```python
from build123d import *

# Parameters (mm, degrees)
F1_DEPTH  = 25.4
F4_SIZE   = 2.286
F5_SIZE   = 3.048
F3_W      = 3.048
F3_H      = 2.286
F6_DEPTH  = 20.066
F7_R      = 8.255
F9_DEPTH  = 25.4
F8_R      = 2.413
F10_DEPTH = 25.4
F11_SIZE  = 1.27
F13_R     = 12.065
F14_DEPTH = 6.35


with BuildPart() as f1:
    # F0 (on Front) → F1 (new body)
    with BuildSketch(Plane.XZ):
        Polygon((18.037553, -0.029708), (9.044504, 15.606125), (-8.993048, 15.635833), (-18.037553, 0.029708), (-9.044504, -15.606125), (8.993048, -15.635833), align=None)
    extrude(amount=F1_DEPTH)

    # F4
    f4_edges = [f1.edges().sort_by_distance(p)[0] for p in [
        (13.541028, 0, 7.788208),
        (0.025728, 0, 15.620979),
        (-13.515301, 0, 7.83277),
        (-13.541028, 0, -7.788208),
        (-0.025728, 0, -15.620979),
        (13.515301, 0, -7.83277),
    ]]
    chamfer(f4_edges, length=F4_SIZE)

    # F5
    f5_edges = [f1.edges().sort_by_distance(p)[0] for p in [
        (13.541028, -25.4, 7.788208),
        (0.025728, -25.4, 15.620979),
        (-13.515301, -25.4, 7.83277),
        (-13.541028, -25.4, -7.788208),
        (-0.025728, -25.4, -15.620979),
        (13.515301, -25.4, -7.83277),
    ]]
    chamfer(f5_edges, length=F5_SIZE)

    # F3 (on offset) → F6 (join)
    with BuildSketch(Plane.XZ.offset(2.286)):
        with Locations((18.87098, 0)):
            Rectangle(F3_W, F3_H)
        Polygon((9.207623, 18.234071), (7.683623, 15.594425), (9.663357, 14.451425), (11.187357, 17.091071), align=None)
        Polygon((-11.187357, 17.091071), (-9.663357, 14.451425), (-7.683623, 15.594425), (-9.207623, 18.234071), align=None)
        with Locations((-18.87098, 0)):
            Rectangle(F3_W, F3_H)
        Polygon((-9.207623, -18.234071), (-7.683623, -15.594425), (-9.663357, -14.451425), (-11.187357, -17.091071), align=None)
        Polygon((11.187357, -17.091071), (9.663357, -14.451425), (7.683623, -15.594425), (9.207623, -18.234071), align=None)
    extrude(amount=F6_DEPTH)

    # F7 (on Front) → F9 (join)
    with BuildSketch(Plane.XZ):
        Circle(F7_R)
    extrude(amount=-F9_DEPTH)

    # F8 (on Front) → F10 (cut)
    with BuildSketch(Plane.XZ):
        Circle(F8_R)
    extrude(amount=-F10_DEPTH, mode=Mode.SUBTRACT)

    # F11
    f11_edges = [f1.edges().sort_by_distance(p)[0] for p in [
        (8.255, 12.7, 0),
        (-8.255, 0, 0),
        (-8.255, 25.4, 0),
    ]]
    chamfer(f11_edges, length=F11_SIZE)

    # F13 (on offset) → F14 (cut)
    with BuildSketch(Plane.XZ.offset(25.4)):
        Circle(F13_R)
    extrude(amount=-F14_DEPTH, mode=Mode.SUBTRACT)


solid = f1.part
```
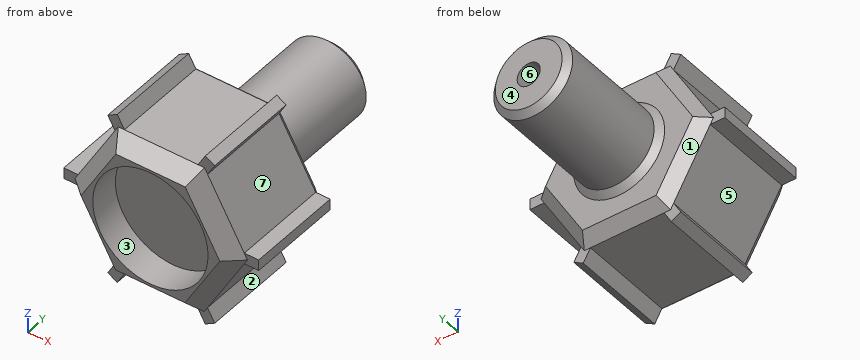
Part model, mm, in its own coordinate system. Face numbers are marked on the shaded views. A direction names the side the tool comes from. Round coordinates to 2 decimals unless told otherwise and drop trailing zeros. Loops run counter-clockwise (first coordinate to the right, second up) from the corner with the lowest first, then second, coordinate; pieces in that order, holes last.
1. Slice it at B-B (x = 0). Give the cut face in (y, z) (3 decimals).
Solutions:
outline: (-25.4, -12.573) - (-22.352, -15.621) - (-2.286, -15.621) - (0, -13.335) - (0, -9.525) - (1.27, -8.255) - (24.13, -8.255) - (25.4, -6.985) - (25.4, -2.413) - (0, -2.413) - (0, 2.413) - (25.4, 2.413) - (25.4, 6.985) - (24.13, 8.255) - (1.27, 8.255) - (0, 9.525) - (0, 13.335) - (-2.286, 15.621) - (-22.352, 15.621) - (-25.4, 12.573) - (-25.4, 12.065) - (-19.05, 12.065) - (-19.05, -12.065) - (-25.4, -12.065) - close
2. Drill centre lines: line 1 along Y through (x, z) = (4, 12); line 2 along Z through (x, y) = (0, 6.5) (3 decimals); line 3 along Y through (x, z) = (1, -3). Where is each one in solid material? Low to high.
Solutions:
line 1: y = -25.4 to 0
line 2: z = -8.255 to -2.413, 2.413 to 8.255
line 3: y = -19.05 to 25.4
3. Two-plate mould, pull along X, no slides. Class the marked faces 1, 2, 3 and 4: pulls with the +X half, pulls with the -X half, needs draft (parallel to the pull), parting line crosses it, or undercut.
Solutions:
face 1: pulls with the -X half
face 2: pulls with the +X half
face 3: undercut
face 4: needs draft
4. Slice it at A-A (y = -20). Give the cut face in (x, z) (3 decimals), and give its area (3 significant figures).
Solutions:
outline: (-20.395, -1.143) - (-17.363, -1.143) - (-9.686, -14.491) - (-11.187, -17.091) - (-9.208, -18.234) - (-7.692, -15.608) - (7.706, -15.634) - (9.208, -18.234) - (11.187, -17.091) - (9.671, -14.465) - (17.392, -1.143) - (20.395, -1.143) - (20.395, 1.143) - (17.363, 1.143) - (9.686, 14.491) - (11.187, 17.091) - (9.208, 18.234) - (7.692, 15.608) - (-7.706, 15.634) - (-9.208, 18.234) - (-11.187, 17.091) - (-9.671, 14.465) - (-17.392, 1.143) - (-20.395, 1.143) - close; hole circle Ø24.13 at (0, 0)
area: 425 mm2
5. Slice it at C-C (y = 11.5). Give the cut face in (x, z) (3 decimals), and give its area (3 significant figures).
Solutions:
outline: circle Ø16.51 at (0, 0); hole circle Ø4.826 at (0, 0)
area: 196 mm2
6. 3-axis set-ups, long thin cutter, end or side, ignore diameter. For the marked faces 5, 6 and 7: which of +Z, -Z, +X, -X, +Y, -Y reach the whole face in a straight line?
Solutions:
face 5: -X, +Y, -Y
face 6: +Y
face 7: +X, +Y, -Y
7. Flat gauge pins, fed straight in: pin 1 (1 mm diameter, centred on x = -10, z = 17, fed in from +Y); pin 2 (1 mm diameter, centred on x = 9, z = 16, fed in from -Y); pin 3 (3 mm diameter, centred on x = 9, z = 17, fed in from +Y). Where does each tip first touch, or does it go through?
Solutions:
pin 1: stops at y = -2.29
pin 2: stops at y = -22.46
pin 3: stops at y = -2.18
